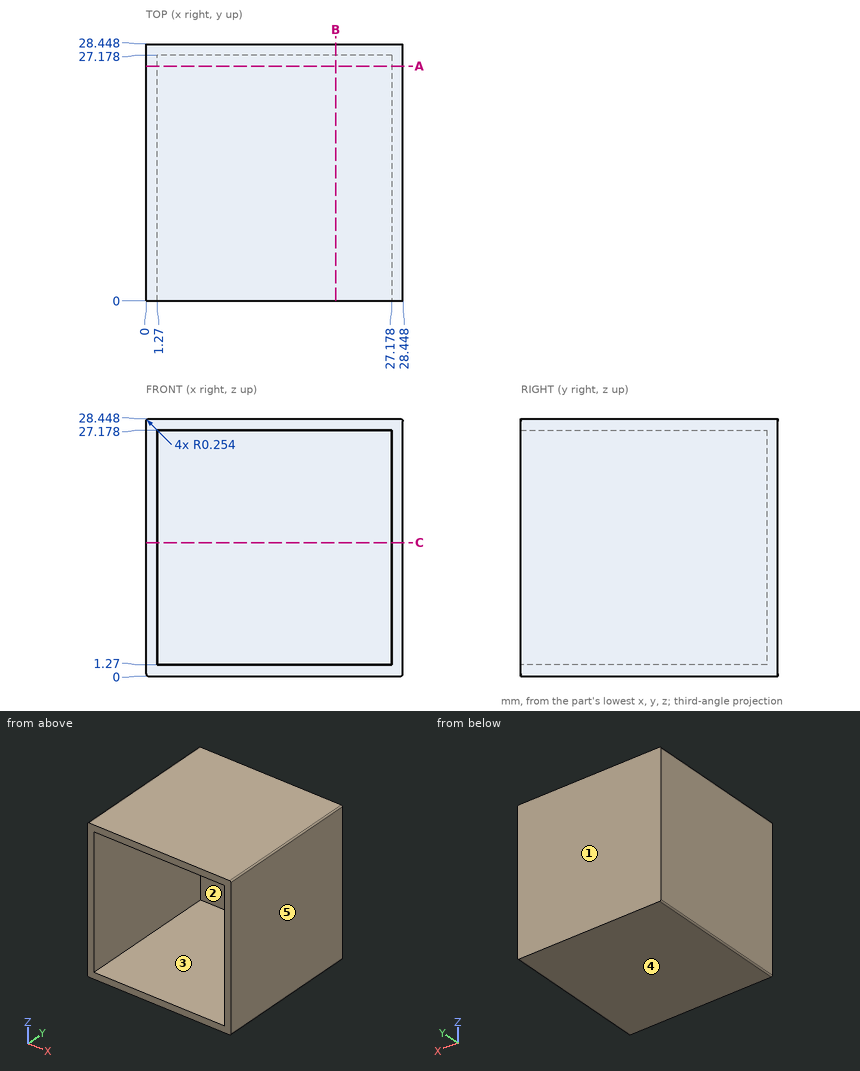
Design review of the part shown in the three views and the two pictorial views. Dimensions are in mm from the part's minimum x, y and z. A direction names the side the tool comes from. Coordinates: 2 decimals unless noted, no trailing zeros. Loops run counter-clockwise (first coordinate to the right, second up) from the corner with the lowest first, then second, coordinate; pieces in that order, holes last. Notation, with made-up numbers: M 25.5,15.25 L 69.5,15.25 A29 cw 69.5,51.25 Z; hole C 19.25,76 d1. An arc over 180 degrees is marked long. Put each result on its own line as item: value. Start each with the question number.
Q1. Add section A-A (y = 26). Write out the cut boundary in (x, z).
Q2. Clearance check with a flat-ended pin moving along its axis: pin 1 (4 mm diameter, centred on x = 3.5, z = 22.5, fed in from -Y). State where the tip first meets the part, or that it passes through.
Q3. Add section C-C (z = 14.75). Write out the cut boundary in (x, y).
Q4. The part is to be moulded in two halves that separate along X. For the marked faces 3, 4 and 5, say which applies: +X half, -X half, draft (parallel to the pull), parting line (faces both ways), or undercut.
Q5. Wall thickness on line 1 (Z direction, x = 3.5, y = 7); line 2 (Y direction, x = 6.25, z = 20.5): over which ranges is each line inside the solid? List them lowest first.
Q6. For the marked faces 1 and 2, list the 3-axis set-ups (+Z, -Z, +X, -X, +Y, -Y) from which the entire face can be reached by the end or side of a thin tool; tool diameter is ignored.
Q7. Add section B-B (x = 21). Write out the cut boundary in (y, z).
Answers:
1. outline: M 0,0.25 A0.25 ccw 0.25,0 L 28.19,0 A0.25 ccw 28.45,0.25 L 28.45,28.19 A0.25 ccw 28.19,28.45 L 0.25,28.45 A0.25 ccw 0,28.19 Z; hole M 1.27,1.27 L 27.18,1.27 L 27.18,27.18 L 1.27,27.18 Z
2. pin 1: stops at y = 27.18
3. outline: M 0,0 L 1.27,0 L 1.27,27.18 L 27.18,27.18 L 27.18,0 L 28.45,0 L 28.45,28.45 L 0,28.45 Z
4. face 3: undercut
4. face 4: draft
4. face 5: +X half
5. line 1: z = 0 to 1.27, 27.18 to 28.45
5. line 2: y = 27.18 to 28.45
6. face 1: +Z, -Z, +X, -X, +Y
6. face 2: -Y
7. outline: M 0,0 L 28.45,0 L 28.45,28.45 L 0,28.45 L 0,27.18 L 27.18,27.18 L 27.18,1.27 L 0,1.27 Z
